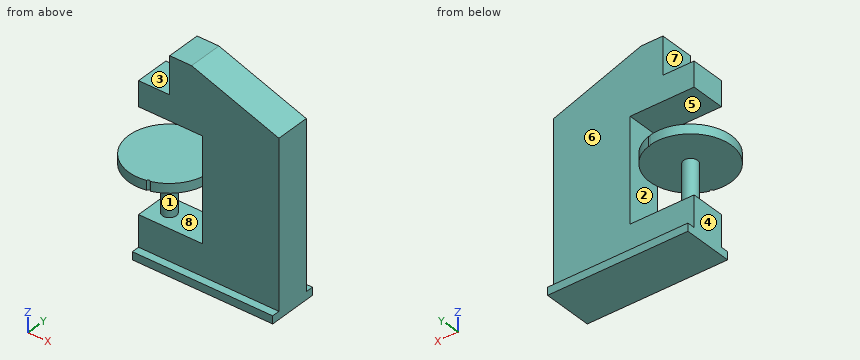
from build123d import *

# Parameters (mm, degrees)
F1_DEPTH = 55
F2_W     = 450
F2_H     = 160
F3_DEPTH = 25
F7_D     = 10


with BuildPart() as f1:
    # F0 (on Front) → F1 (new body, symmetric)
    with BuildSketch(Plane.XZ):
        Polygon((0, 125), (0, 0), (450, 0), (450, 555), (170, 655), (100, 655), (100, 535), (0, 535), (0, 455), (205, 455), (205, 125), align=None)
    extrude(amount=F1_DEPTH, both=True)

    # F2 (on Top) → F3 (join)
    with BuildSketch(Plane.XY):
        with Locations((225, 0)):
            Rectangle(F2_W, F2_H)
    extrude(amount=F3_DEPTH)

    # F4 (on Front) → F5 (revolve)
    with BuildSketch(Plane.XZ):
        Polygon((32.5, 275), (32.5, 125), (55, 125), (55, 305), (-75, 305), (-75, 275), align=None)
    revolve(axis=Axis((55, 0, 215), (0, 0, -1)))

    # F7 (through all)
    with Locations(Plane(origin=(0, 0, 0), x_dir=(1, 0, 0), z_dir=(0, 0, -1))):
        with Locations((88.3679986, 126.6223043203), (602.5738120079, 126.6223043203), (602.5738120079, -128.7268400192), (88.3679986, -128.7268400192)):
            Hole(F7_D / 2)


solid = f1.part
CAD build for the part. Positions are in the model's coordinates, mm. Face numbers are marked on the shaded views. A direction names the side the tool comes from. Round coordinates to 2 decimals unless told otherwise and drop trailing zeros. Order: outer loops, then holes, each group sorted by start corner. A loop starts at its lowest first (then second) coordinate and runs counter-clockwise, first axis right, second up. Notation, with made-up numbers: (-35.5, 32.25) - (6.5, 32.25) arc R27 cw to (6.5, 68.25) - close; hole circle Ø9 at (65.25, 86). An arc over 180 degrees is marked (long way). Return JSON: item names as keys, results as strings.
(1) Pin check, flat tips, straight feed: pin 1 Ø3 at (x, z) = (71, 97.5) entering from -Y; pin 2 Ø4 at (x, y) = (72.5, -55) entering from +Z; pin 3 Ø20 at (x, y) = (192, 73.5) entering from +Z. Stop position of each tip, or through.
Answer key:
{"pin 1": "stops at y = -55", "pin 2": "stops at z = 535", "pin 3": "stops at z = 25"}
(2) Cut at A-A (x = 55). Give the cut face in (y, z), then the cut area to 4 significant figures.
Answer key:
{"outline": "(-130, 275) - (-22.5, 275) - (-22.5, 125) - (-55, 125) - (-55, 25) - (-80, 25) - (-80, 0) - (80, 0) - (80, 25) - (55, 25) - (55, 125) - (22.5, 125) - (22.5, 275) - (130, 275) - (130, 305) - (-130, 305) - close; (-55, 455) - (55, 455) - (55, 535) - (-55, 535) - close", "area": "38,350 mm^2"}
(3) Cut at C-C (z = 361). Give the cut face in (x, y).
Answer key:
{"outline": "(205, -55) - (450, -55) - (450, 55) - (205, 55) - close"}
(4) Cut at D-D (x = 413.5). Give the cut face in (y, z), then the cut area to 3 significant figures.
Answer key:
{"outline": "(-80, 0) - (80, 0) - (80, 25) - (55, 25) - (55, 568.04) - (-55, 568.04) - (-55, 25) - (-80, 25) - close", "area": "63,700 mm^2"}
(5) Wall check: probe 1 along Z at (x, y) = (142, -76); probe 2 along Y at (x, z) = (354, 177.5); probe 3 along X at (y, z) = (-33.5, 336.5). Give the ranges that are in metal, low to high. Write a range as from..to.
Answer key:
{"probe 1": "z = 0..25, 275..305", "probe 2": "y = -55..55", "probe 3": "x = 205..450"}
(6) Tool access for the marked faces 1, 2, 3, 4 and 5: list every direction of +Z, -Z, +X, -X, +Y, -Y with a clear straight run to the whole face (end or side of a thin tool).
Answer key:
{"face 1": "none", "face 2": "+Y, -Y", "face 3": "+Z, -X, +Y, -Y", "face 4": "-Z, -X, +Y, -Y", "face 5": "-X, +Y, -Y"}
(7) Pull direction X, two halves, no side cores. Call the marked faces 6, 7 and 8: +X half, -X half, draft (parallel to the pull), parting line (faces both ways), or undercut.
Answer key:
{"face 6": "draft", "face 7": "-X half", "face 8": "undercut"}
(8) Cut at B-B (y = 0). Give the cut face in (x, z), then the cut area to 3 significant figures.
Answer key:
{"outline": "(-75, 275) - (32.5, 275) - (32.5, 125) - (0, 125) - (0, 0) - (450, 0) - (450, 555) - (170, 655) - (100, 655) - (100, 535) - (0, 535) - (0, 455) - (205, 455) - (205, 125) - (77.5, 125) - (77.5, 275) - (185, 275) - (185, 305) - (-75, 305) - close", "area": "216,000 mm^2"}
